from build123d import *

# Parameters (mm, degrees)
F1_DEPTH = 10
F3_DEPTH = 14
F5_DEPTH = 12


with BuildPart() as f1:
    # F0 (on Front) → F1 (new body, symmetric)
    with BuildSketch(Plane.XZ):
        with BuildLine():
            ThreePointArc((12.787234, -15.378122), (0, -20), (-12.787234, -15.378122))
            ThreePointArc((-12.787234, -15.378122), (-17.716171, -15.831528), (-17.262766, -20.760465))
            ThreePointArc((-17.262766, -20.760465), (0, -27), (17.262766, -20.760465))
            ThreePointArc((17.262766, -20.760465), (17.716171, -15.831528), (12.787234, -15.378122))
        make_face()
        with BuildLine():
            ThreePointArc((-13.525, -18.069294), (-13.606362, -18.556598), (-13.841621, -18.991038))
            ThreePointArc((-13.841621, -18.991038), (-16.443638, -17.581989), (-13.525, -18.069294))
        make_face(mode=Mode.SUBTRACT)
        with BuildLine():
            ThreePointArc((16.525, -18.069294), (15.512304, -19.487932), (13.841621, -18.991038))
            ThreePointArc((13.841621, -18.991038), (14.537696, -16.650655), (16.525, -18.069294))
        make_face(mode=Mode.SUBTRACT)
    extrude(amount=F1_DEPTH, both=True)

    # F2 (on face) → F3 (cut)
    with BuildSketch(Plane.XZ.offset(10)):
        with BuildLine():
            Line((31.764954, -10.083012), (-3.385311, -12.986047))
            Line((-3.385311, -12.986047), (-5.867412, -19.119976))
            ThreePointArc((-5.867412, -19.119976), (3.933364, -19.609402), (12.787234, -15.378122))
            ThreePointArc((12.787234, -15.378122), (17.716171, -15.831528), (17.262766, -20.760465))
            ThreePointArc((17.262766, -20.760465), (5.011502, -26.530828), (-8.500477, -25.626976))
            Line((-8.500477, -25.626976), (-10.211368, -29.855039))
            Line((-10.211368, -29.855039), (28.234236, -31.502709))
            Line((28.234236, -31.502709), (31.764954, -10.083012))
        make_face()
        with BuildLine():
            ThreePointArc((12.787234, -15.378122), (3.933364, -19.609402), (-5.867412, -19.119976))
            Line((-5.867412, -19.119976), (-8.500477, -25.626976))
            ThreePointArc((-8.500477, -25.626976), (5.011502, -26.530828), (17.262766, -20.760465))
            ThreePointArc((17.262766, -20.760465), (17.716171, -15.831528), (12.787234, -15.378122))
        make_face()
        with BuildLine():
            ThreePointArc((13.841621, -18.991038), (14.537696, -16.650655), (16.525, -18.069294))
            ThreePointArc((16.525, -18.069294), (15.512304, -19.487932), (13.841621, -18.991038))
        make_face(mode=Mode.SUBTRACT)
    extrude(amount=-F3_DEPTH, mode=Mode.SUBTRACT)

    # F4 (on face) → F5 (cut)
    with BuildSketch(Plane(origin=(0, 10, 0), x_dir=(-1, 0, 0), z_dir=(0, 1, 0))):
        Polygon((7.364115, -14.344795), (13.547452, -27.560162), (28.157102, -12.950514), align=None)
    extrude(amount=-F5_DEPTH, mode=Mode.SUBTRACT)


solid = f1.part
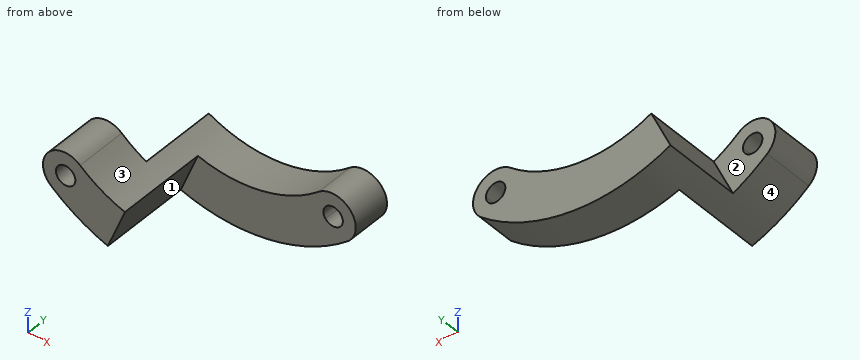
Geometry check sheet. Reference: the model listing, model coordinates, mm. Face numbers are marked on the shaded views. Give positions to 0.01 mm unless a question says otherwise; leave off trailing zeros. Write each loop counter-clockwise with the first axis right and the second up, starting at its lowest first coordinate (ties: lowest second). Pieces come first, ordered by that corner, then holes. Notation, with made-up numbers: (82.25, -25) - (109.25, -25) arc R29 ccw to (109.25, -2) - close; hole circle Ø6 at (34.5, 86.5). An arc over 180 degrees is marked (long way). Put each result on its own line as item: value.
1. Thickness scan on line 1 (X direction, y = 6, z = -18.5); line 2 (Y direction, x = 4.5, z = -22); line 3 (X direction, y = -2.75, z = -17.5). Record the ranges inside material, lowest first.
Ans:
line 1: x = -9.31 to -7.6, 7.6 to 13.59, 16.46 to 18.5
line 2: y = 4 to 10
line 3: x = -18.48 to -16.41, -13.64 to -9.68
2. Go/stop test with flat-tipped pins: pin 1 (6 mm diameter, centred on y = 3, z = -18, fed in from -X); pin 2 (2 mm diameter, centred on x = -12, y = -2, fed in from +Z); pin 3 (1.5 mm diameter, centred on x = -4.5, z = -19, fed in from -Y). Record where each tip stops, or that it passes through.
Ans:
pin 1: stops at x = -10.48
pin 2: stops at z = -15.21
pin 3: stops at y = 4
3. Sectioned sample at B-B, the plane x = 14.5. Enter the section's corners in (y, z).
Ans:
outline: (4, -22.78) - (10, -22.78) - (10, -19.47) - (4, -19.47) - close; (4, -16.66) - (10, -16.66) - (10, -14.61) - (4, -14.61) - close
4. Draft check along X on the marked faces 1, 2, 3 and 4. Enter one of: +X half, -X half, draft (parallel to the pull), parting line (faces both ways), or undercut.
Ans:
face 1: +X half
face 2: draft
face 3: undercut
face 4: parting line
5. Sectioned sample at D-D, the plane z = -23. Enter the section's corners in (x, y).
Ans:
outline: (-14.14, -10) - (-7.44, -10) - (-7.44, 4) - (14.14, 4) - (14.14, 10) - (-11.41, 10) - (-11.41, -2) - (-14.14, -2) - close
6. Sectioned sample at C-C, the plane z = -18.5. Enter the section's corners in (x, y), plus the area to 3 significant figures.
Ans:
outline: (-18.5, -10) - (-16.46, -10) - (-16.46, -2) - (-18.5, -2) - close; (-13.59, -10) - (-7.6, -10) - (-7.6, 10) - (-9.31, 10) - (-9.31, -2) - (-13.59, -2) - close; (7.6, 4) - (13.59, 4) - (13.59, 10) - (7.6, 10) - close; (16.46, 4) - (18.5, 4) - (18.5, 10) - (16.46, 10) - close
area: 133 mm²
7. Sectioned sample at A-A, the plane y = 7.5. Enter the section's corners in (x, z) (3 decimals), plus the area to 3 significant figures.
Ans:
outline: (-11.975, -24.199) arc R27 ccw to (17.263, -20.76) arc R3.5 ccw to (12.787, -15.378) arc R20 cw to (-9.007, -17.857) - close; hole circle Ø3 at (15.025, -18.069)
area: 202 mm²
